Autodesk Inventor part; units mm, degrees
ref_plane "YZ Plane" through (0, 0, 0) normal (1, 0, 0) x (0, 1, 0)
ref_plane "XZ Plane" through (0, 0, 0) normal (0, 1, 0) x (-1, 0, 0)
ref_plane "XY Plane" through (0, 0, 0) normal (0, 0, 1) x (1, 0, 0)
sketch "Sketch1" plane through (0, 0, 0) normal (0, 0, 1) x (1, 0, 0)
  circle A0 centre (190, 3.5) radius 5.5
  circle A1 centre (-192, 668.25) radius 5.5
  arc A2 (176.9945, -3.9737) -> (203.0055, 10.9737) centre (190, 3.5) ccw
  arc A3 (-178.9945, 675.7237) -> (-205.0055, 660.7763) centre (-192, 668.25) ccw
  circle A4 centre (190, 3.5) radius 5.5
  circle A5 centre (-192, 668.25) radius 5.5
  line L0 (-178.9945, 675.7237) -> (203.0055, 10.9737)
  line L1 (176.9945, -3.9737) -> (-205.0055, 660.7763)
  point P0 (0, 0)
  dimension "d2" = 11
  dimension "d3" = 30
  dimension "d4" = 11
  dimension "d5" = 30
extrude "Extrusion2" add sketch "Sketch1" along normal blind 6
properties part number "90-08-1550" material "Steel, Mild"
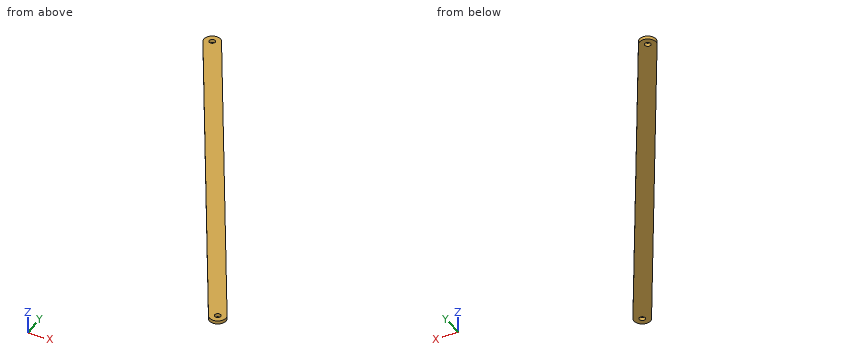
Geometry: final body of the model. Coordinates: model frame, mm. Give positions to 0.01 mm unless a question says otherwise; leave off trailing zeros. Write each loop counter-clockwise with the first axis right and the second up, starting at its lowest first coordinate (ties: lowest second). Pieces come first, ordered by that corner, then holes. Notation, with made-up numbers: M 85.5,64.5 L 108.5,64.5 A18 cw 108.5,74.5 Z; hole C 14.5,-23 d8. An arc over 180 degrees is marked long. Answer in a Markdown table with one row per item. Add a question column.
(1) Section A-A on z = 3.75. Return loops of the section in (x, y).
(2) Ray query, line 1 (X direction, y = 668.25, z = 4.3); line 2 (Y direction, x = 190, z = 3.15); line 3 (Y direction, x = -192, z = 3.45). Return the intervals inside material, ascending.
(3) Section C-C on y = 327. Return loops of the section in (x, z).
(4) First-contact query: pin 1 (2 mm diameter, centred on x = 125, z = 1, fed in from -Y); pin 2 (1 mm diameter, centred on y = 218.5, z = 2.5, fed in from +X); pin 3 (1 mm diameter, centred on x = 70.5, z = 2, fed in from +Y). Flat tips, straight axial feed; report the tip coordinate or a pass-through.
(5) Section B-B on x = 168.5. Return loops of the section in (y, z).
Result set:
| question | item | result |
|---|---|---|
| 1 | outline | M -205.01,660.78 L 176.99,-3.97 A15 ccw 203.01,10.97 L -178.99,675.72 A15 ccw Z; hole C -192,668.25 d11; hole C 190,3.5 d11 |
| 2 | line 1 | x = -207 to -197.5, -186.5 to -174.7 |
| 2 | line 2 | y = -11.5 to -2, 9 to 33.61 |
| 2 | line 3 | y = 638.14 to 662.75, 673.75 to 683.25 |
| 3 | outline | M -13.2,0 L 21.4,0 L 21.4,6 L -13.2,6 Z |
| 4 | pin 1 | stops at y = 84.77 |
| 4 | pin 2 | stops at x = 84.04 |
| 4 | pin 3 | stops at y = 242.43 |
| 5 | outline | M 10.81,0 L 71.02,0 L 71.02,6 L 10.81,6 Z |
